```python
from build123d import *

# Parameters (mm, degrees)
SKETCH1_R               = 50
BOSS_EXTRUDE1_DEPTH     = 5
SKETCH2_R               = 2.5
BOSS_EXTRUDE2_DEPTH     = 30
BOSS_EXTRUDE3_OUTLINE_R = 50
BOSS_EXTRUDE3_DEPTH     = 30
SKETCH4_R               = 39
CUT_EXTRUDE1_DEPTH      = 6


# Read off the part's stored shape, not the designer's step: Boss-Extrude3
with BuildPart() as part:
    # Sketch1 → Boss-Extrude1 (new body)
    with BuildSketch(Plane(origin=(0, 0, 0), x_dir=(1, 0, 0), z_dir=(0, 1, 0))):
        with Locations(Location((0, 0, 0), (0, 0, 270))):
            Circle(SKETCH1_R)
    extrude(amount=BOSS_EXTRUDE1_DEPTH)

    # Sketch2 → Boss-Extrude2 (add)
    with BuildSketch(Plane(origin=(0, 5, 0), x_dir=(1, 0, 0), z_dir=(0, 1, 0))):
        with Locations(Location((43, 0, 0), (0, 0, 270))):
            Circle(SKETCH2_R)
        with Locations(Location((36.173901912, -23.247555151, 0), (0, 0, 270))):
            Circle(SKETCH2_R)
        with Locations(Location((17.862845559, -39.1141758, 0), (0, 0, 270))):
            Circle(SKETCH2_R)
        with Locations(Location((-6.119538046, -42.562322001, 0), (0, 0, 270))):
            Circle(SKETCH2_R)
        with Locations(Location((-28.15901156, -32.497231697, 0), (0, 0, 270))):
            Circle(SKETCH2_R)
        with Locations(Location((-41.258197865, -12.114499944, 0), (0, 0, 270))):
            Circle(SKETCH2_R)
        with Locations(Location((-41.258197865, 12.114499944, 0), (0, 0, 270))):
            Circle(SKETCH2_R)
        with Locations(Location((-28.15901156, 32.497231697, 0), (0, 0, 270))):
            Circle(SKETCH2_R)
        with Locations(Location((-6.119538046, 42.562322001, 0), (0, 0, 270))):
            Circle(SKETCH2_R)
        with Locations(Location((17.862845559, 39.1141758, 0), (0, 0, 270))):
            Circle(SKETCH2_R)
        with Locations(Location((36.173901912, 23.247555151, 0), (0, 0, 270))):
            Circle(SKETCH2_R)
    extrude(amount=BOSS_EXTRUDE2_DEPTH)

    # Boss-Extrude3 outline → Boss-Extrude3 (add)
    with BuildSketch(Plane(origin=(0, 5, 0), x_dir=(1, 0, 0), z_dir=(0, 1, 0))):
        Circle(BOSS_EXTRUDE3_OUTLINE_R)
        with BuildLine():
            ThreePointArc((45.686046512, 5.365179786), (49, 0), (45.686046512, -5.365179786))
            ThreePointArc((45.686046512, -5.365179786), (44.136676786, -12.959697615), (41.334183214, -20.186265083))
            ThreePointArc((41.334183214, -20.186265083), (41.221423109, -26.491400055), (35.532912844, -29.213217982))
            ThreePointArc((35.532912844, -29.213217982), (30.123593761, -34.76448042), (23.8590088, -39.328713418))
            ThreePointArc((23.8590088, -39.328713418), (20.355335637, -44.571967772), (14.098330411, -43.786265879))
            ThreePointArc((14.098330411, -43.786265879), (6.54648256, -45.531786327), (-1.191232329, -45.984573126))
            ThreePointArc((-1.191232329, -45.984573126), (-6.973427076, -48.501250652), (-11.812372312, -44.457483738))
            ThreePointArc((-11.812372312, -44.457483738), (-19.109090598, -41.843071786), (-25.86326561, -38.040655778))
            ThreePointArc((-25.86326561, -38.040655778), (-32.088175963, -37.031729143), (-33.972730289, -31.013764633))
            ThreePointArc((-33.972730289, -31.013764633), (-38.69766251, -24.869477603), (-42.323894801, -18.019099003))
            ThreePointArc((-42.323894801, -18.019099003), (-47.015155707, -13.804895285), (-45.346986439, -7.723394389))
            ThreePointArc((-45.346986439, -7.723394389), (-46, 0), (-45.346986439, 7.723394389))
            ThreePointArc((-45.346986439, 7.723394389), (-47.015155707, 13.804895285), (-42.323894801, 18.019099003))
            ThreePointArc((-42.323894801, 18.019099003), (-38.69766251, 24.869477603), (-33.972730289, 31.013764633))
            ThreePointArc((-33.972730289, 31.013764633), (-32.088175963, 37.031729143), (-25.86326561, 38.040655778))
            ThreePointArc((-25.86326561, 38.040655778), (-19.109090598, 41.843071786), (-11.812372312, 44.457483738))
            ThreePointArc((-11.812372312, 44.457483738), (-6.973427076, 48.501250652), (-1.191232329, 45.984573126))
            ThreePointArc((-1.191232329, 45.984573126), (6.54648256, 45.531786327), (14.098330411, 43.786265879))
            ThreePointArc((14.098330411, 43.786265879), (20.355335637, 44.571967772), (23.8590088, 39.328713418))
            ThreePointArc((23.8590088, 39.328713418), (30.123593761, 34.76448042), (35.532912844, 29.213217982))
            ThreePointArc((35.532912844, 29.213217982), (41.221423109, 26.491400055), (41.334183214, 20.186265083))
            ThreePointArc((41.334183214, 20.186265083), (44.136676786, 12.959697615), (45.686046512, 5.365179786))
        make_face(mode=Mode.SUBTRACT)
    extrude(amount=BOSS_EXTRUDE3_DEPTH)

    # Sketch4 → Cut-Extrude1 (cut)
    with BuildSketch(Plane(origin=(0, 5, 0), x_dir=(1, 0, 0), z_dir=(0, 1, 0))):
        with Locations(Location((0, 0, 0), (0, 0, 270))):
            Circle(SKETCH4_R)
    extrude(amount=-CUT_EXTRUDE1_DEPTH, mode=Mode.SUBTRACT)


solid = part.part
```
Read the model definition and answer for the solid it produces. Units are mm, in the model's axes. A direction names the side the tool comes from. Round coordinates to 2 decimals unless told otherwise and drop trailing zeros. Write each loop counter-clockwise with the first axis right and the second up, starting at its lowest first coordinate (ties: lowest second). Pieces come first, ordered by that corner, then holes. Notation, with made-up numbers: (-23.75, 84) -> (25.25, 84) arc R11 cw to (25.25, 92) -> close; hole circle Ø3 at (34.5, -23.5). An arc over 180 degrees is marked (long way). Answer in a Markdown table with one row per item. Add a question column.
1) Given P1, Ø5, axis at y = 31.5, z = -27, coming from the +X side; P2, Ø1, axis at x = 13, y = 17.5, coming from the +Z side; P3, Ø1.5, axis at x = -4.5, z = 39.5, coming from the -Y side; P4, Ø3, axis at y = 27, z = -30, coming from the +X side, each flat-ended and moving along its own axis, determine where each tip first touches the part or whether it passes through.
2) Consider line 1 (Z direction, x = 0.5, y = 9.5); line 2 (X direction, y = 3, z = 0); line 3 (X direction, y = 27, z = -31). Determine where each line is inside the solid, lowest interval first.
3) Which of the six approach directions +Z, -Z, +X, -X, +Y, -Y give full straight-line access (tool end or side, diameter ignored) to faces 1 (the face through (40.56, 19.79, -0.54)), 2 (the face through (38.668, 2.535, -5.077))?
4) Find section A-A, the plane x = -13. Determine the outline of the cut face in (y, z).
5) Find section B-B, the plane y = 23.5. State how many separate pieces and enclosed holes the cut face has, and give its area (3 significant figures).
6) Determine the mould class of faces 3 (the face through (20.44, 19.79, 44.533)), 4 (the face through (36, 35, 23)) for opening direction X: pulls with the +X half, pulls with the -X half, needs draft (parallel to the pull), parting line crosses it, or undercut.
Findings below:
| question | item | result |
|---|---|---|
| 1 | P1 | x = 43.59 |
| 1 | P2 | z = 48.41 |
| 1 | P3 | y = 0 |
| 1 | P4 | x = 41.08 |
| 2 | line 1 | -50 to -46, 46 to 50 |
| 2 | line 2 | -50 to -39, 39 to 50 |
| 2 | line 3 | -39.23 to -33.99, -30.16 to -26.16, 33.99 to 39.23 |
| 3 | face 1 | +Y |
| 3 | face 2 | +Y, -Y |
| 4 | outline | (0, -48.28) -> (35, -48.28) -> (35, -44.12) -> (5, -44.12) -> (5, -36.77) -> (0, -36.77) -> close; (0, 36.77) -> (5, 36.77) -> (5, 44.12) -> (35, 44.12) -> (35, 48.28) -> (0, 48.28) -> close |
| 5 | separate pieces | 12 |
| 5 | enclosed holes | 1 |
| 5 | area | 1,170 mm² |
| 6 | face 3 | undercut |
| 6 | face 4 | needs draft |
